The model under review builds one solid part; all positions refer to its coordinate system, in mm. Face numbers are marked on the shaded views. Round coordinates to 2 decimals unless told otherwise and drop trailing zeros. Order: outer loops, then holes, each group sorted by start corner. A loop starts at its lowest first (then second) coordinate and runs counter-clockwise, first axis right, second up. Notation, with made-up numbers: (15, 6) -> (69, 6) arc R28 ccw to (69, 28) -> close; hole circle Ø1 at (65.25, 49.25). An arc over 180 degrees is marked (long way). Use a Markdown table: item, result. Add a question column.
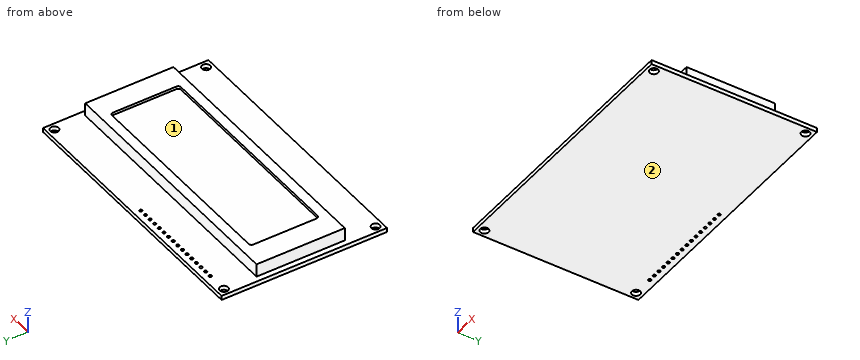
```python
from build123d import *

# Parameters (mm, degrees)
ESQUISSE1_W             = 98
ESQUISSE1_H             = 60
ESQUISSE1_R             = 1.5
ESQUISSE1_R_2           = 0.5
BOSS_EXTRU_1_DEPTH      = 1.55
ESQUISSE2_W             = 94
ESQUISSE2_H             = 32
BOSS_EXTRU_2_DEPTH      = 4.75
ENL_V_MAT_EXTRU_2_DEPTH = 1


with BuildPart() as part:
    # Esquisse1 → Boss.-Extru.1 (new body)
    with BuildSketch(Plane.XY):
        with Locations((-13.900836029, 1.990498339)):
            Rectangle(ESQUISSE1_W, ESQUISSE1_H)
        with Locations(Location((-60.400836029, 29.490498339, 0), (0, 0, 180))):
            Circle(ESQUISSE1_R, mode=Mode.SUBTRACT)
        with Locations(Location((32.599163971, 29.490498339, 0), (0, 0, 180))):
            Circle(ESQUISSE1_R, mode=Mode.SUBTRACT)
        with Locations(Location((32.599163971, -25.509501661, 0), (0, 0, 180))):
            Circle(ESQUISSE1_R, mode=Mode.SUBTRACT)
        with Locations(Location((-60.400836029, -25.509501661, 0), (0, 0, 180))):
            Circle(ESQUISSE1_R, mode=Mode.SUBTRACT)
        with Locations((-52.900836029, 29.490498339)):
            Circle(ESQUISSE1_R_2, mode=Mode.SUBTRACT)
        with Locations((-50.360836029, 29.490498339)):
            Circle(ESQUISSE1_R_2, mode=Mode.SUBTRACT)
        with Locations((-47.820836029, 29.490498339)):
            Circle(ESQUISSE1_R_2, mode=Mode.SUBTRACT)
        with Locations((-45.280836029, 29.490498339)):
            Circle(ESQUISSE1_R_2, mode=Mode.SUBTRACT)
        with Locations((-42.740836029, 29.490498339)):
            Circle(ESQUISSE1_R_2, mode=Mode.SUBTRACT)
        with Locations((-40.200836029, 29.490498339)):
            Circle(ESQUISSE1_R_2, mode=Mode.SUBTRACT)
        with Locations((-37.660836029, 29.490498339)):
            Circle(ESQUISSE1_R_2, mode=Mode.SUBTRACT)
        with Locations((-35.120836029, 29.490498339)):
            Circle(ESQUISSE1_R_2, mode=Mode.SUBTRACT)
        with Locations((-32.580836029, 29.490498339)):
            Circle(ESQUISSE1_R_2, mode=Mode.SUBTRACT)
        with Locations((-30.040836029, 29.490498339)):
            Circle(ESQUISSE1_R_2, mode=Mode.SUBTRACT)
        with Locations((-27.500836029, 29.490498339)):
            Circle(ESQUISSE1_R_2, mode=Mode.SUBTRACT)
        with Locations((-24.960836029, 29.490498339)):
            Circle(ESQUISSE1_R_2, mode=Mode.SUBTRACT)
        with Locations((-22.420836029, 29.490498339)):
            Circle(ESQUISSE1_R_2, mode=Mode.SUBTRACT)
        with Locations((-19.880836029, 29.490498339)):
            Circle(ESQUISSE1_R_2, mode=Mode.SUBTRACT)
        with Locations((-17.340836029, 29.490498339)):
            Circle(ESQUISSE1_R_2, mode=Mode.SUBTRACT)
        with Locations((-14.800836029, 29.490498339)):
            Circle(ESQUISSE1_R_2, mode=Mode.SUBTRACT)
    extrude(amount=BOSS_EXTRU_1_DEPTH)

    # Esquisse2 → Boss.-Extru.2 (add)
    with BuildSketch(Plane.XY.offset(1.55)):
        with Locations((-13.900836029, 1.990498339)):
            Rectangle(ESQUISSE2_W, ESQUISSE2_H)
    extrude(amount=BOSS_EXTRU_2_DEPTH)

    # Esquisse5 → Enlèv. mat.-Extru.2 (cut)
    with BuildSketch(Plane.XY.offset(6.3)):
        with BuildLine():
            Line((-51.300836029, 14.490498339), (23.699163971, 14.490498339))
            ThreePointArc((23.699163971, 14.490498339), (24.406270752, 14.19760512), (24.699163971, 13.490498339))
            Line((24.699163971, 13.490498339), (24.699163971, -9.509501661))
            ThreePointArc((24.699163971, -9.509501661), (24.406270752, -10.216608442), (23.699163971, -10.509501661))
            Line((23.699163971, -10.509501661), (-51.300836029, -10.509501661))
            ThreePointArc((-51.300836029, -10.509501661), (-52.00794281, -10.216608442), (-52.300836029, -9.509501661))
            Line((-52.300836029, -9.509501661), (-52.300836029, 13.490498339))
            ThreePointArc((-52.300836029, 13.490498339), (-52.00794281, 14.19760512), (-51.300836029, 14.490498339))
        make_face()
    extrude(amount=-ENL_V_MAT_EXTRU_2_DEPTH, mode=Mode.SUBTRACT)


solid = part.part
```
Q1. Draft analysis for pull direction X (two halves, no side actions). For the marked faces 1 and 2, state which applies: released by +X, released by -X, zero draft, split by the parting line, or undercut.
Q2. Add section D-D, the plane y = -18.5. Give the boundary of the cut face in (x, z), then the cut area to 3 significant figures.
Q3. To check wall thickness, follow line 1 along Y through (x, z) = (6, 5.5); line 2 along Y through (x, z) = (-37, 3.75); line 3 along Z through (x, y) = (18, 27). State the ranges of each line that lie inside material, in increasing order.
Q4. Add section C-C, the plane z = 2.5. Give the boundary of the cut face in (x, y).
Q5. Add section A-A, the plane x = 6. Give the boundary of the cut face in (y, z).
Q6. For pin 1 (1.4 mm diameter, centred on y = -6, z = 3.5, fed in from -X); pin 2 (2.5 mm diameter, centred on x = -60.4, y = 29.49, fed in from -Z); pin 3 (10 mm diameter, centred on x = -9, y = -3, fed in from +Z); pin 4 (5 mm diameter, centred on x = -60.4, y = -25.51, fed in from +Z), all flat-tipped, find the tip position at first contact; note any pin that passes through.
Q7. Add section B-B, the plane y = -12. Give the boundary of the cut face in (x, z).
Return value:
| question | item | result |
|---|---|---|
| 1 | face 1 | undercut |
| 1 | face 2 | zero draft |
| 2 | outline | (-62.9, 0) -> (35.1, 0) -> (35.1, 1.55) -> (-62.9, 1.55) -> close |
| 2 | area | 152 mm² |
| 3 | line 1 | -14.01 to -10.51, 14.49 to 17.99 |
| 3 | line 2 | -14.01 to 17.99 |
| 3 | line 3 | 0 to 1.55 |
| 4 | outline | (-60.9, -14.01) -> (33.1, -14.01) -> (33.1, 17.99) -> (-60.9, 17.99) -> close |
| 5 | outline | (-28.01, 0) -> (31.99, 0) -> (31.99, 1.55) -> (17.99, 1.55) -> (17.99, 6.3) -> (14.49, 6.3) -> (14.49, 5.3) -> (-10.51, 5.3) -> (-10.51, 6.3) -> (-14.01, 6.3) -> (-14.01, 1.55) -> (-28.01, 1.55) -> close |
| 6 | pin 1 | x = -60.9 |
| 6 | pin 2 | through |
| 6 | pin 3 | z = 5.3 |
| 6 | pin 4 | z = 1.55 |
| 7 | outline | (-62.9, 0) -> (35.1, 0) -> (35.1, 1.55) -> (33.1, 1.55) -> (33.1, 6.3) -> (-60.9, 6.3) -> (-60.9, 1.55) -> (-62.9, 1.55) -> close |
